Read the model definition and answer for the solid it produces. Units are mm, in the model's axes. A direction names the side the tool comes from. Coordinates: 2 decimals unless noted, no trailing zeros. Order: outer loops, then holes, each group sorted by start corner. A loop starts at its lowest first (then second) coordinate and runs counter-clockwise, first axis right, second up.
from build123d import *

# Parameters (mm, degrees)
BOSS_EXTRUDE2_DEPTH = 80
SKETCH8_W           = 20
SKETCH8_H           = 20
CUT_EXTRUDE5_DEPTH  = 205
SKETCH9_W           = 30
SKETCH9_H           = 60
CUT_EXTRUDE6_DEPTH  = 205
SKETCH10_W          = 20
SKETCH10_H          = 20
CUT_EXTRUDE8_DEPTH  = 150
SKETCH13_R          = 10
CUT_EXTRUDE9_DEPTH  = 150
BOSS_EXTRUDE5_DEPTH = 40
CUT_EXTRUDE10_DEPTH = 20
CUT_EXTRUDE15_DEPTH = 20
SKETCH18_W          = 10
SKETCH18_H          = 20
CUT_EXTRUDE16_DEPTH = 0.0001


with BuildPart() as part:
    # Sketch1 → Boss-Extrude2 (new body)
    with BuildSketch(Plane.XY):
        with BuildLine():
            ThreePointArc((80, 20), (60, 0), (80, -20))
            Line((80, -20), (90, -20))
            Line((90, -20), (90, -50))
            Line((90, -50), (0, -50))
            ThreePointArc((0, -50), (-50, 0), (0, 50))
            Line((0, 50), (90, 50))
            Line((90, 50), (90, 20))
            Line((90, 20), (80, 20))
        make_face()
    extrude(amount=BOSS_EXTRUDE2_DEPTH)

    # Sketch8 → Cut-Extrude5 (cut)
    with BuildSketch(Plane(origin=(90, 0, 0), x_dir=(0, 0, -1), z_dir=(1, 0, 0))):
        with Locations((-10, 40)):
            Rectangle(SKETCH8_W, SKETCH8_H)
    extrude(amount=-CUT_EXTRUDE5_DEPTH, mode=Mode.SUBTRACT)

    # Sketch9 → Cut-Extrude6 (cut)
    with BuildSketch(Plane(origin=(-50, 0, 0), x_dir=(0, 0, -1), z_dir=(1, 0, 0))):
        with Locations((-65, 0)):
            Rectangle(SKETCH9_W, SKETCH9_H)
    extrude(amount=CUT_EXTRUDE6_DEPTH, mode=Mode.SUBTRACT)

    # Sketch10 → Cut-Extrude8 (cut)
    with BuildSketch(Plane(origin=(90, 0, 0), x_dir=(0, 0, -1), z_dir=(1, 0, 0))):
        with Locations((-70, 40)):
            Rectangle(SKETCH10_W, SKETCH10_H)
    extrude(amount=-CUT_EXTRUDE8_DEPTH, mode=Mode.SUBTRACT)

    # Sketch13 → Cut-Extrude9 (cut)
    with BuildSketch(Plane.XY.offset(50)):
        Circle(SKETCH13_R)
    extrude(amount=-CUT_EXTRUDE9_DEPTH, mode=Mode.SUBTRACT)

    # Sketch14 → Boss-Extrude5 (add)
    with BuildSketch(Plane(origin=(0, 0, 0), x_dir=(-1, 0, 0), z_dir=(0, 0, -1))):
        with BuildLine():
            Line((-80, 20), (-80, -20))
            ThreePointArc((-80, -20), (-60, 0), (-80, 20))
        make_face()
    extrude(amount=-BOSS_EXTRUDE5_DEPTH)

    # Sketch15 → Cut-Extrude10 (cut)
    with BuildSketch(Plane(origin=(0, 0, 0), x_dir=(-1, 0, 0), z_dir=(0, 0, -1))):
        with BuildLine():
            Line((-80, 20), (-80, -20))
            ThreePointArc((-80, -20), (-60, 0), (-80, 20))
        make_face()
    extrude(amount=-CUT_EXTRUDE10_DEPTH, mode=Mode.SUBTRACT)

    # Sketch16 → Cut-Extrude15 (cut)
    with BuildSketch(Plane(origin=(0, 0, 0), x_dir=(-1, 0, 0), z_dir=(0, 0, -1))):
        with BuildLine():
            Line((-10, 0), (-49.99900001, 0))
            ThreePointArc((-49.99900001, 0), (-35.354985511, -35.354278404), (-0.001, -49.999))
            Line((-0.001, -49.999), (-0.001, -9.99999995))
            ThreePointArc((-0.001, -9.99999995), (-7.071421356, -7.07071425), (-10, 0))
        make_face()
        with BuildLine():
            Line((-0.001, 30), (-40, 30))
            ThreePointArc((-40, 30), (-47.434164903, 15.811388301), (-50, 0))
            Line((-50, 0), (-49.99900001, 0))
            Line((-49.99900001, 0), (-10, 0))
            ThreePointArc((-10, 0), (-7.071421356, 7.07071425), (-0.001, 9.99999995))
            Line((-0.001, 10), (-0.001, 30))
        make_face()
    extrude(amount=-CUT_EXTRUDE15_DEPTH, mode=Mode.SUBTRACT)

    # Sketch18 → Cut-Extrude16 (cut)
    with BuildSketch(Plane(origin=(0, -50, 0), x_dir=(-1, 0, 0), z_dir=(0, -1, 0))):
        with Locations((-5, -10)):
            Rectangle(SKETCH18_W, SKETCH18_H)
    extrude(amount=-CUT_EXTRUDE16_DEPTH, mode=Mode.SUBTRACT)


solid = part.part
Q1. Which of the six approach directions +Z, -Z, +X, -X, +Y, -Y give full straight-line access (tool end or side, diameter ignored) to faces 4 (the cylindrical face through (47.362, 16.025, 9.86)), 5 (the flat face through (85, 20, 25)), 6 (the flat face through (19, 0, 50))?
Q2. The part is cut by section C-C, the plane x = -26.5. Determine the outline of the cut face in (y, z).
Q3. Determine the mould class of faces 1 (the flat face through (90, 35, 36)), 2 (the flat face through (46, -50, 39)), 3 (the flat face through (0.001, 20, 10)) for opening direction X: +X half, -X half, draft (parallel to the pull), parting line (faces both ways), or undercut.
Q4. The part is cut by section A-A, the plane z = 55.5. Determine the outline of the cut face in (x, y), then the cut area to 3 significant figures.
Q5. Straight lines are drawn through the part: L1, parallel to Y at x = 19.5, z = 55; L2, parallel to Y at x = 0, z = 36; L3, parallel to X at y = 0, z = 26. For each, find the intervals that lie inside material, in ascending order.
Q6. The part is cut by section B-B, the plane z = 37.5. Determine the outline of the cut face in (x, y), then the cut area to 3 significant figures.
Q7. Each of these flat-tipped pins is pushed along its axis until it touches: P1, Ø22, axis at x = 69, z = 7.5, coming from the +Y side; P2, Ø16, axis at x = 68.5, y = 3, coming from the -Z side; P3, Ø4, axis at x = 29.5, z = 65.5, coming from the +Y side; P4, Ø10, axis at y = 17.5, z = 9, coming from the +X side. Where does it stop, or does it pass through?
Computed values:
1. face 4: -Z
1. face 5: +Z, -Z, +X
1. face 6: +Z, +X, -X
2. outline: (-42.4, 0) - (30, 0) - (30, 20) - (42.4, 20) - (42.4, 60) - (30, 60) - (30, 50) - (-30, 50) - (-30, 80) - (-42.4, 80) - close
3. face 1: +X half
3. face 2: draft
3. face 3: undercut
4. outline: (-40, -30) arc R50 ccw to (0, -50) - (90, -50) - (90, -30) - close; (-40, 30) - (90, 30) - (90, 50) - (0, 50) arc R50 ccw to start
4. area: 4,720 mm2
5. L1: y = -50 to -30, 30 to 50
5. L2: y = -50 to -10, 10 to 50
5. L3: x = -50 to -10, 10 to 80
6. outline: (0, -50) - (90, -50) - (90, -20) - (80, -20) - (80, 20) - (90, 20) - (90, 50) - (0, 50) arc R50 ccw to start; hole circle Ø20 at (0, 0)
6. area: 12,200 mm2
7. P1: stops at y = 30
7. P2: stops at z = 20
7. P3: stops at y = -30
7. P4: stops at x = 90
